Source: three-view drawing plus pictorial views. Frame: mm from the lowest corner of the part. Coordinates: 2 decimals unless noted, no trailing zeros. Loops run counter-clockwise (first coordinate to the right, second up) from the corner with the lowest first, then second, coordinate; pieces in that order, holes last. Notation, with made-up numbers: M 17,-24 L 43,-24 A35 ccw 43,10 Z; hole C 79,83.5 d1. An arc over 180 degrees is marked long. Use a Markdown table: item, result. Add a question column.
1. Section D-D on z = 33. Output: boundary loops of the cut face in (x, y).
2. Section A-A on y = 21. Output: boundary loops of the cut face in (x, z).
3. Section C-C on x = 19. Output: boundary loops of the cut face in (y, z), then the cut area to 3 significant figures.
4. Line query: L1, parallel to X at y = 5.5, z = 40.5; L2, parallel to Y at x = 29.5, z = 30.5; L3, parallel to Z at x = 41, y = 21.5. Output: solid intervals per line, ascending. Write a range as [from, to].
5. Pin query (flat end, axial travel): pin 1 (3.5 mm diameter, centred on y = 2, z = 13.5, fed in from +X); pin 2 (6.5 mm diameter, centred on x = 41, y = 12, fed in from -Z); pin 3 (1 mm diameter, centred on x = 11.5, z = 19.5, fed in from +Y). Return the tip coordinate at first contact, or that it passes through.
6. Section B-B on y = 16.25. Output: boundary loops of the cut face in (x, z).
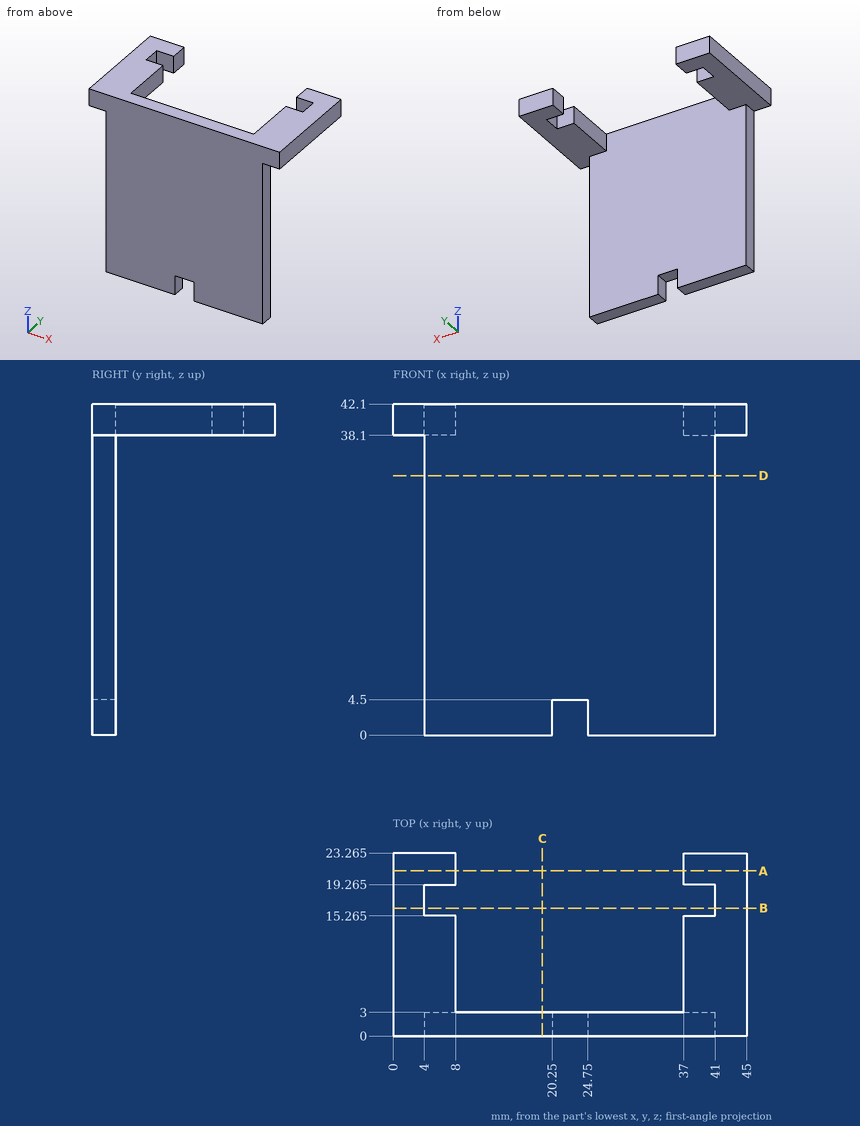
Answers below:
| question | item | result |
|---|---|---|
| 1 | outline | M 4,0 L 41,0 L 41,3 L 4,3 Z |
| 2 | outline | M 0,38.1 L 8,38.1 L 8,42.1 L 0,42.1 Z; M 37,38.1 L 45,38.1 L 45,42.1 L 37,42.1 Z |
| 3 | outline | M 0,0 L 3,0 L 3,42.1 L 0,42.1 Z |
| 3 | area | 126 mm² |
| 4 | L1 | x = [0, 8], [37, 45] |
| 4 | L2 | y = [0, 3] |
| 4 | L3 | z = [38.1, 42.1] |
| 5 | pin 1 | stops at x = 41 |
| 5 | pin 2 | stops at z = 38.1 |
| 5 | pin 3 | stops at y = 3 |
| 6 | outline | M 0,38.1 L 4,38.1 L 4,42.1 L 0,42.1 Z; M 41,38.1 L 45,38.1 L 45,42.1 L 41,42.1 Z |
